```python
from build123d import *

# Parameters (mm, degrees)
SKETCH1_W               = 25.4
SKETCH1_H               = 12.7
SKETCH1_H_2             = 63.5
BOSS_EXTRUDE1_DEPTH     = 33.3756
CUT_EXTRUDE2_DEPTH      = 57.663045059
CUT_EXTRUDE2_DEPTH_BACK = 57.663045059
SKETCH5_R               = 3.175
CUT_EXTRUDE3_DEPTH      = 6.35
BOSS_EXTRUDE2_REACH     = 63.744
SKETCH1_5_W             = 25.4
SKETCH1_5_H             = 12.7
SKETCH7_W               = 25.4
SKETCH7_H               = 3.175
BOSS_EXTRUDE3_DEPTH     = 12.7
FILLET1_R               = 6.35


with BuildPart() as part:
    # Sketch1 → Boss-Extrude1 (new body)
    with BuildSketch(Plane(origin=(0, 0, 0), x_dir=(1, 0, 0), z_dir=(0, 1, 0))):
        with Locations((0, -31.75)):
            Rectangle(SKETCH1_W, SKETCH1_H)
        with Locations((0, 6.35)):
            Rectangle(SKETCH1_W, SKETCH1_H_2)
    extrude(amount=BOSS_EXTRUDE1_DEPTH)

    # Sketch4 → Cut-Extrude2 (cut, two sides: drawn at the far end of the back side and taken through both)
    with BuildSketch(Plane(origin=(12.7, 0, 0), x_dir=(0, 0, -1), z_dir=(1, 0, 0)).offset(-CUT_EXTRUDE2_DEPTH_BACK)):
        Polygon((38.1, 33.3756), (-38.1, 33.3756), (-38.1, 7.879436654), align=None)
    extrude(amount=CUT_EXTRUDE2_DEPTH + CUT_EXTRUDE2_DEPTH_BACK, mode=Mode.SUBTRACT)

    # Sketch5 → Cut-Extrude3 (cut)
    with BuildSketch(Plane(origin=(0, 18.550693474, 6.20697521), x_dir=(1, 0, 0), z_dir=(0, 0.9483236552061992, 0.3173046564050927))):
        with Locations(Location((0, 6.545207615, 0), (0, 0, 270))):
            Circle(SKETCH5_R)
    extrude(amount=-CUT_EXTRUDE3_DEPTH, mode=Mode.SUBTRACT)

    # Boss-Extrude2: from a plane face, 63.744 long prism both ways, kept between that surface and its translate by the depth
    boss_extrude2_start = Plane(origin=(-12.7, 7.879436654, 38.1), z_dir=(0, -0.9483236552061992, -0.3173046564050927)) * Box(256.976, 256.976, 128.488, align=(Align.CENTER, Align.CENTER, Align.MIN), mode=Mode.PRIVATE)
    boss_extrude2_end = Plane(origin=(-12.7, 17.404436654, 38.1), z_dir=(0, -0.9483236552061992, -0.3173046564050927)) * Box(256.976, 256.976, 128.488, align=(Align.CENTER, Align.CENTER, Align.MIN), mode=Mode.PRIVATE)
    # Sketch1_5 → Boss-Extrude2 (add, from a surface)
    with BuildSketch(Plane(origin=(0, 0, 0), x_dir=(1, 0, 0), z_dir=(0, 1, 0)), mode=Mode.PRIVATE) as boss_extrude2_sk1:
        with Locations((0, -31.75)):
            Rectangle(SKETCH1_5_W, SKETCH1_5_H)
    boss_extrude2_tool1 = extrude(boss_extrude2_sk1.sketch, amount=BOSS_EXTRUDE2_REACH, both=True, mode=Mode.PRIVATE)
    add(((boss_extrude2_tool1 - boss_extrude2_start) & boss_extrude2_end).solids().sort_by_distance((0, 16.891297, 31.75))[0])

    # Sketch7 → Boss-Extrude3 (add, along a direction that is not the sketch's normal)
    with BuildSketch(Plane(origin=(0, 0, 25.4), x_dir=(-1, 0, 0), z_dir=(0, 0, -1))):
        with Locations((0, 20.066297212)):
            Rectangle(SKETCH7_W, SKETCH7_H)
    extrude(amount=BOSS_EXTRUDE3_DEPTH, dir=(0, 0.31730465640509264, -0.9483236552061991))

    # Fillet1
    fillet1_edges = [part.edges().sort_by_distance(p)[0] for p in [
        (-12.7, 16.6878, -38.1),
        (-12.7, 8.702218327, 38.1),
        (12.7, 16.6878, -38.1),
        (12.7, 8.702218327, 38.1),
    ]]
    fillet(fillet1_edges, radius=FILLET1_R)


solid = part.part
```
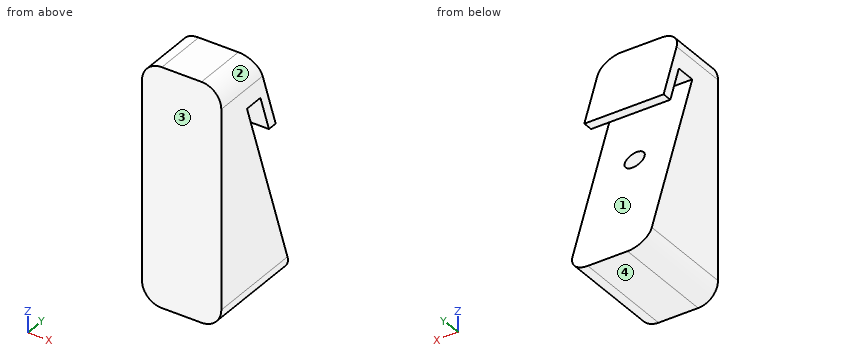
Read the model definition and answer for the solid it produces. Units are mm, in the model's axes. Face numbers are marked on the shaded views. Round coordinates to 2 decimals unless told otherwise and drop trailing zeros. Write each loop counter-clockwise with the first axis right and the second up, starting at its lowest first coordinate (ties: lowest second). Pieces come first, ordered by that corner, then holes. Notation, with made-up numbers: (-37, -2.75) -> (14, -2.75) arc R32 cw to (14, 36.25) -> close; hole circle Ø3 at (-18, 82.25). An arc over 180 degrees is marked (long way). Answer in a Markdown table with one row per item. Add a question column.
1) Given P1, Ø12, axis at x = -5.5, z = 0, coming from the +Y side; P2, Ø2, axis at x = -10, z = 1.5, coming from the +Y side; P3, Ø5, axis at x = 8.5, z = -19, coming from the +Y side, each flat-ended and moving along its own axis, determine where each tip first touches the part or whether it passes through.
2) Find section D-D, the plane x = -1.75. Determine the outline of the cut face in (y, z).
3) Find section C-C, the plane z = -13.5. Determine the outline of the cut face in (x, y), and give its area (3 significant figures).
4) Find section A-A, the plane x = 4.5. Determine the outline of the cut face in (y, z).
5) Find section B-B, the plane y = 7. Determine the outline of the cut face in (x, z), and give its area (3 significant figures).
6) Consider line 1 (X direction, y = 16, z = -4.5); line 2 (Y direction, x = 7, z = 22); line 3 (Y direction, x = 9.5, z = 15). Determine where each line is inside the solid, lowest interval first.
7) Determine the mould class of the marked faces 1, 2, 3 and 4 for opening direction Z: pulls with the +Z half, pulls with the -Z half, needs draft (parallel to the pull), parting line crosses it, or undercut.
Findings below:
| question | item | result |
|---|---|---|
| 1 | P1 | y = 22.64 |
| 1 | P2 | y = 20.46 |
| 1 | P3 | y = 27.82 |
| 2 | outline | (0, -38.1) -> (33.38, -38.1) -> (21.47, -2.51) -> (15.45, -4.53) -> (13.77, 0.5) -> (19.79, 2.51) -> (12.13, 25.4) -> (18.48, 25.4) -> (22.51, 13.36) -> (25.68, 13.36) -> (17.4, 38.1) -> (0, 38.1) -> close |
| 3 | outline | (-12.7, 0) -> (12.7, 0) -> (12.7, 25.14) -> (-12.7, 25.14) -> close |
| 3 | area | 639 mm² |
| 4 | outline | (0, -38.1) -> (33.38, -38.1) -> (12.13, 25.4) -> (18.48, 25.4) -> (22.51, 13.36) -> (25.68, 13.36) -> (17.4, 38.1) -> (0, 38.1) -> close |
| 5 | outline | (-12.7, -31.75) arc R6.35 ccw to (-6.35, -38.1) -> (6.35, -38.1) arc R6.35 ccw to (12.7, -31.75) -> (12.7, 31.75) arc R6.35 ccw to (6.35, 38.1) -> (-6.35, 38.1) arc R6.35 ccw to (-12.7, 31.75) -> close |
| 5 | area | 1,900 mm² |
| 6 | line 1 | -12.7 to -1.5, 1.5 to 12.7 |
| 6 | line 2 | 0 to 13.27, 19.62 to 22.79 |
| 6 | line 3 | 0 to 15.61, 21.96 to 25.13 |
| 7 | face 1 | undercut |
| 7 | face 2 | pulls with the +Z half |
| 7 | face 3 | needs draft |
| 7 | face 4 | pulls with the -Z half |
